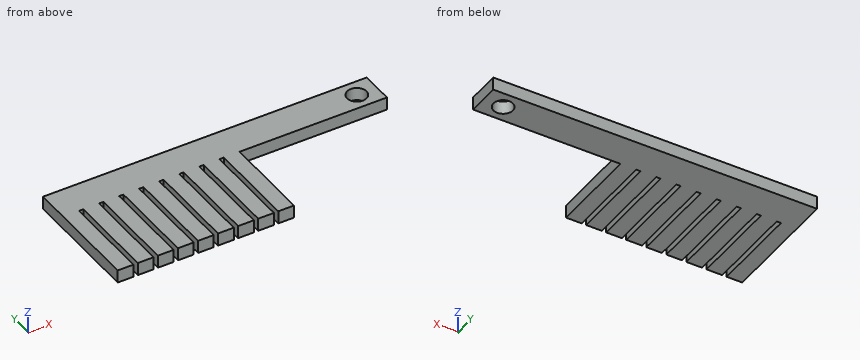
```python
from build123d import *

# Parameters (mm, degrees)
F0_W     = 6.16181
F0_H     = 34.9758
F1_DEPTH = 5.08
F2_R     = 3.81
F3_DEPTH = 25.4


with BuildPart() as f1:
    # F0 (on Top) → F1 (new body)
    with BuildSketch(Plane.XY):
        Polygon((-111.135946, 33.877251), (-111.135946, 20.877251), (-104.974136, 20.877251), (-103.261946, 20.877251), (-97.100136, 20.877251), (-95.387946, 20.877251), (-89.226136, 20.877251), (-87.513946, 20.877251), (-81.352136, 20.877251), (-79.639946, 20.877251), (-73.478136, 20.877251), (-71.765946, 20.877251), (-65.604136, 20.877251), (-63.891946, 20.877251), (-57.730136, 20.877251), (-56.017946, 20.877251), (-49.856136, 20.877251), (-48.143946, 20.877251), (-41.982136, 20.877251), (15.864054, 20.877251), (15.864054, 33.877251), align=None)
        with Locations((-108.055041, 3.389351)):
            Rectangle(F0_W, F0_H)
        with Locations((-100.181041, 3.389351)):
            Rectangle(F0_W, F0_H)
        with Locations((-92.307041, 3.389351)):
            Rectangle(F0_W, F0_H)
        with Locations((-45.063041, 3.389351)):
            Rectangle(F0_W, F0_H)
        with Locations((-84.433041, 3.389351)):
            Rectangle(F0_W, F0_H)
        with Locations((-52.937041, 3.389351)):
            Rectangle(F0_W, F0_H)
        with Locations((-76.559041, 3.389351)):
            Rectangle(F0_W, F0_H)
        with Locations((-60.811041, 3.389351)):
            Rectangle(F0_W, F0_H)
        with Locations((-68.685041, 3.389351)):
            Rectangle(F0_W, F0_H)
    extrude(amount=F1_DEPTH)

    # F2 (on face) → F3 (cut)
    with BuildSketch(Plane.XY.offset(5.08)):
        with Locations((8.004281, 27.377251)):
            Circle(F2_R)
    extrude(amount=-F3_DEPTH, mode=Mode.SUBTRACT)


solid = f1.part
```
Part model, mm, in its own coordinate system. Coordinates: 2 decimals unless noted, no trailing zeros. Write each loop counter-clockwise with the first axis right and the second up, starting at its lowest first coordinate (ties: lowest second). Pieces come first, ordered by that corner, then holes.
Item 1: Probe line 1 (Y direction, x = -19, z = 2.1); line 2 (X direction, y = 30, z = 0.8). List the from-to ranges inside material, lowest first.
Item 2: Pin check, flat tips, straight feed: pin 1 (1.9 mm diameter, centred on x = -48.5, z = 1.5, fed in from -Y); pin 2 (2.5 mm diameter, centred on y = 3, z = 2.5, fed in from +X); pin 3 (0.5 mm diameter, centred on x = -57, z = 2.5, fed in from -Y). Stop position of each tip, or through.
Item 3: Slice it at A-A (x = -26.5). Write the cut outline in (y, z), and give its area (3 significant figures).
Item 4: Slice it at B-B (y = -8). Count the separate pieces of the cut face and the enclosed holes in it, and give its area (3 significant figures).
Results found:
1. line 1: y = 20.88 to 33.88
1. line 2: x = -111.14 to 5.24, 10.77 to 15.86
2. pin 1: stops at y = -14.1
2. pin 2: stops at x = -41.98
2. pin 3: stops at y = 20.88
3. outline: (20.88, 0) - (33.88, 0) - (33.88, 5.08) - (20.88, 5.08) - close
3. area: 66.0 mm2
4. separate pieces: 9
4. enclosed holes: 0
4. area: 282 mm2
